For this review, take the finished solid that the model builds, in its own axes (mm). Give positions to 0.01 mm unless a question says otherwise; leave off trailing zeros. Write each loop counter-clockwise with the first axis right and the second up, starting at its lowest first coordinate (ties: lowest second). Pieces come first, ordered by that corner, then holes. Notation, with made-up numbers: M 15,-30.75 L 38,-30.75 A15 cw 38,-13.75 Z; hole C 51.5,-4 d9. An arc over 180 degrees is marked long. Answer as a JSON object with one key per item and string values. Group by question number.
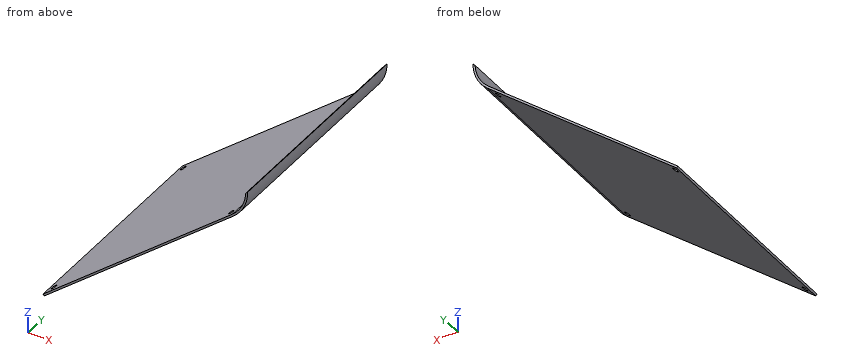
Autodesk Inventor part; units mm, degrees
ref_plane "YZ Plane" through (0, 0, 0) normal (1, 0, 0) x (0, 1, 0)
ref_plane "XZ Plane" through (0, 0, 0) normal (0, 1, 0) x (-1, 0, 0)
ref_plane "XY Plane" through (0, 0, 0) normal (0, 0, 1) x (1, 0, 0)
sketch "Sketch1" plane through (0, 0, 0) normal (0, 1, 0) x (-1, 0, 0)
  line L0 (131.6241, -133.8819) -> (133.2116, -133.8819)
  arc A0 (0, 0) -> (11.8436, -25.4008) centre (33.1555, -0.0022) ccw
  line L1 (11.8436, -25.4008) -> (167.5038, -156.0152)
  arc A1 (1.5875, 0) -> (1.5875, -0.0044) centre (33.1555, -0.0022) ccw
  line L2 (12.864, -24.1847) -> (168.5242, -154.7991)
  line L3 (168.5242, -154.7991) -> (167.5038, -156.0152)
  line L4 (0, -0.0044) -> (1.6297, -1.6341)
  arc A2 (1.6297, -1.6341) -> (12.864, -24.1847) centre (33.1555, -0.0022) ccw
  dimension "d15" = 1.5875
extrude "Extrusion1" add sketch "Sketch1" along normal blind 177.8
sketch "Sketch2" plane through (-12.864, 0, -24.1847) normal (-0.6427876, 0, 0.7660444) x (0.7660444, 0, 0.6427876)
  line L0 (0, 0) -> (0, 177.8)
  line L1 (-203.2, 0) -> (-185.2395, 0) construction
  line L2 (0, 165.1) -> (17.9605, 165.1) construction
  line L3 (-203.2, 165.1) -> (-185.2395, 165.1) construction
  point P0 (25.4, 0)
  point P1 (-6.35, 6.35)
  point P2 (-196.85, 6.35)
  point P3 (-203.2, 177.8)
  point P4 (-6.35, 171.45)
  point P5 (-196.85, 171.45)
hole "Hole1" at (-163.6598, 6.35, -150.7174) at (-163.6598, 171.45, -150.7174) at (-17.7284, 171.45, -28.2664) at (-17.7284, 6.35, -28.2664) direction (0.6427876, 0, -0.7660444) diameter 4.7625 end through all
properties part number "intakeabs" material "Polyethylene, High Density"
Item 1: Consider section A-A (y = 48). Give the boundary of the cut face in (x, z).
Item 2: Consider section B-B (z = -66). Give the boundary of the cut face in (x, y), plus the area to 3 significant figures.
Item 3: To check wall thickness, follow probe 1 along X at (y, z) = (85.5, -127); probe 2 along Z at (x, y) = (-149, 123.5); probe 3 along Z at (x, y) = (-77, 140). State the ranges of each line that lie inside material, in increasing order.
Item 4: Insertion check: P1, Ø10, axis at y = 91, z = -31, coming from the -X side; P2, Ø1.5, axis at x = -57, y = 78.5, coming from the -Z side; P3, Ø1.5, axis at x = -39, y = 78, coming from the -Z side. Each pin has a flat end and moves straight along its axis. Give the tip position at first contact, or say it passes through.
Item 5: Consider section C-C (x = -52). Give the boundary of the cut face in (y, z), plus the area to 3 significant figures.
Result set:
{
 "1": {"outline": "M -168.52,-154.8 L -167.5,-156.02 L -11.84,-25.4 A33.16 ccw 0,0 L -1.63,-1.63 A31.57 cw -12.86,-24.18 Z"},
 "2": {"outline": "M -62.7,0 L -60.23,0 L -60.23,177.8 L -62.7,177.8 Z", "area": "439 mm^2"},
 "3": {"probe 1": "x = -135.39 to -132.92", "probe 2": "z = -140.49 to -138.42", "probe 3": "z = -80.07 to -78"},
 "4": {"P1": "stops at x = -26.94", "P2": "stops at z = -63.92", "P3": "stops at z = -48.82"},
 "5": {"outline": "M 0,-59.1 L 177.8,-59.1 L 177.8,-57.02 L 0,-57.02 Z", "area": "368 mm^2"}
}
